Autodesk Inventor part; units mm, degrees
ref_plane "YZ Plane" through (0, 0, 0) normal (1, 0, 0) x (0, 1, 0)
ref_plane "XZ Plane" through (0, 0, 0) normal (0, 1, 0) x (-1, 0, 0)
ref_plane "XY Plane" through (0, 0, 0) normal (0, 0, 1) x (1, 0, 0)
sketch "Sketch1" plane through (0, 0, 0) normal (0, 1, 0) x (-1, 0, 0)
  line L0 (0, -5.65) -> (0, -36.65)
  line L1 (36.65, -42.3) -> (5.65, -42.3)
  line L2 (42.3, -36.65) -> (42.3, -5.65)
  line L3 (5.65, 0) -> (36.65, 0)
  line L4 (36.65, 0) -> (42.3, -5.65)
  line L5 (42.3, -36.65) -> (36.65, -42.3)
  line L6 (5.65, -42.3) -> (0, -36.65)
  line L7 (0, -5.65) -> (5.65, 0)
  line L8 (5.65, -36.65) -> (36.65, -36.65) construction
  line L9 (36.65, -36.65) -> (36.65, -5.65) construction
  line L10 (36.65, -5.65) -> (5.65, -5.65) construction
  line L11 (5.65, -5.65) -> (5.65, -36.65) construction
  line L12 (5.65, -36.65) -> (36.65, -5.65) construction
  line L13 (36.65, -36.65) -> (5.65, -5.65) construction
  circle A0 centre (36.65, -5.65) radius 1.5
  circle A1 centre (36.65, -36.65) radius 1.5
  circle A2 centre (5.65, -36.65) radius 1.5
  circle A3 centre (5.65, -5.65) radius 1.5
  point P0 (0, 0)
  point P1 (21.15, -21.15)
  dimension "d12" = 3
  dimension "d14" = 3
  dimension "d15" = 3
extrude "Extrusion1" add sketch "Sketch1" along normal blind 34
sketch "Sketch2" plane through (0, 34, 0) normal (0, 1, 0) x (1, 0, 0)
  line L0 (-42.3, 5.65) -> (-36.65, 0) construction
  line L1 (-39.475, 2.825) -> (-2.825, 39.475) construction
  line L2 (0, 36.65) -> (-5.65, 42.3) construction
  line L3 (-36.65, 42.3) -> (-42.3, 36.65) construction
  line L4 (-39.475, 39.475) -> (-2.825, 2.825) construction
  line L5 (-5.65, 0) -> (0, 5.65) construction
  circle A0 centre (-21.15, 21.15) radius 11
  point P0 (0, 0)
  dimension "d18" = 22
extrude "Extrusion2" add sketch "Sketch2" along normal blind 2
sketch "Sketch3" plane through (-21.15, 36, -21.15) normal (0, 1, 0) x (1, 0, 0)
  line L0 (-21.15, -15.5) -> (-15.5, -21.15) construction
  line L1 (-18.325, -18.325) -> (18.325, 18.325) construction
  line L2 (21.15, 15.5) -> (15.5, 21.15) construction
  line L3 (-18.325, 18.325) -> (18.325, -18.325) construction
  line L4 (15.5, -21.15) -> (21.15, -15.5) construction
  circle A0 centre (0, 0) radius 2.5
  point P0 (21.15, -21.15)
  dimension "d21" = 5
extrude "Extrusion3" add sketch "Sketch3" along normal blind 22
properties part number "NEMA16 Motor" material "Steel"
Geometry: final body of the model. Coordinates: model frame, mm. A direction names the side the tool comes from. Round coordinates to 2 decimals unless told otherwise and drop trailing zeros. Write each loop counter-clockwise with the first axis right and the second up, starting at its lowest first coordinate (ties: lowest second). Pieces come first, ordered by that corner, then holes. Notation, with made-up numbers: (24, -21) -> (37, -21) arc R14 cw to (37, -12) -> close; hole circle Ø9 at (75, 38). An arc over 180 degrees is marked (long way). Use CSV: the item, a comma, the result in double quotes. Start each with the question number.
Q1. Section D-D (y = 46). Return loops of the section in (x, z).
Q2. Section B-B (y = 13). Return loops of the section in (x, z).
Q3. Section C-C (z = -21.15). Return loops of the section in (x, y), plus the area to 3 significant figures.
Q4. Section A-A (x = -21.15). Return loops of the section in (y, z).
Q5. Line query: L1, parallel to Z at x = -36.65, y = 12.5; L2, parallel to Z at x = -36, y = 8. Output: solid intervals per line, ascending.
Q6. Reachability of faces 4 (the face through (-38.08, 16.76, -6.1)), 5 (the face through (-32.14, 34.99, -20.67)) from +Z, -Z, +X, -X, +Y, -Y: full face, straight path, thin tool, end or side. Return the list, or none.
Q7. Pull-direction query (Z, two-part tool) for faces 1 (the face through (-21, 58, -21)), 2 (the face through (-2.79, 16.76, -2.86)), 3 (the face through (-5, 17, -7)); classes: pulls with the +Z half, pulls with the -Z half, needs draft (parallel to the pull), parting line crosses it, or undercut.
Q8. First-contact query: pin 1 Ø2 at (x, y) = (-32, 17) entering from +Z; pin 2 Ø5 at (x, z) = (-12, -33.5) entering from +Y. Flat tips, straight axial feed; report the tip coordinate or a pass-through.
Result sheet:
1,outline,"circle Ø5 at (-21.15, -21.15)"
2,outline,"(-42.3, -36.65) -> (-36.65, -42.3) -> (-5.65, -42.3) -> (0, -36.65) -> (0, -5.65) -> (-5.65, 0) -> (-36.65, 0) -> (-42.3, -5.65) -> close; hole circle Ø3 at (-36.65, -36.65); hole circle Ø3 at (-36.65, -5.65); hole circle Ø3 at (-5.65, -36.65); hole circle Ø3 at (-5.65, -5.65)"
3,outline,"(-42.3, 0) -> (0, 0) -> (0, 34) -> (-10.15, 34) -> (-10.15, 36) -> (-18.65, 36) -> (-18.65, 58) -> (-23.65, 58) -> (-23.65, 36) -> (-32.15, 36) -> (-32.15, 34) -> (-42.3, 34) -> close"
3,area,"1,590 mm²"
4,outline,"(0, -42.3) -> (34, -42.3) -> (34, -32.15) -> (36, -32.15) -> (36, -23.65) -> (58, -23.65) -> (58, -18.65) -> (36, -18.65) -> (36, -10.15) -> (34, -10.15) -> (34, 0) -> (0, 0) -> close"
5,L1,"-42.3 to -38.15, -35.15 to -7.15, -4.15 to 0"
5,L2,"-42.3 to -38, -35.3 to -7, -4.3 to 0"
6,face 4,"+Y, -Y"
6,face 5,"+Y"
7,face 1,"needs draft"
7,face 2,"pulls with the +Z half"
7,face 3,"undercut"
8,pin 1,"z = 0"
8,pin 2,"y = 34"
